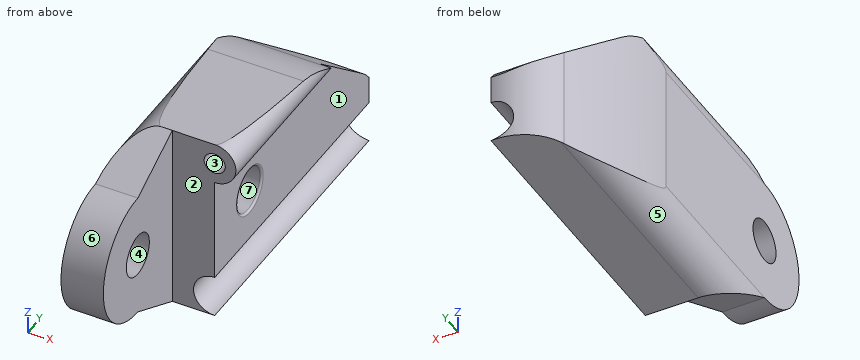
```python
from build123d import *

# Parameters (mm, degrees)
BOSS_EXTRUDE1_DEPTH = 50.8
CUT_EXTRUDE2_START  = -21.59
SKETCH3_R           = 1.27
CUT_EXTRUDE2_DEPTH  = 50.8
CUT_EXTRUDE1_DEPTH  = 50.8
SKETCH4_W           = 10.16
SKETCH4_H           = 15.24
CUT_EXTRUDE3_DEPTH  = 50.8
SKETCH5_R           = 2.54
CUT_EXTRUDE5_DEPTH  = 50.8
CUT_EXTRUDE6_DEPTH  = 32.512
CUT_EXTRUDE7_DEPTH  = 32.512
CUT_EXTRUDE12_START = -10.16
SKETCH14_R          = 2.7
CUT_EXTRUDE12_DEPTH = 9.08
CUT_EXTRUDE9_DEPTH  = 38.608
BOSS_EXTRUDE2_START = -4.2
SKETCH15_R          = 2.7
BOSS_EXTRUDE2_DEPTH = 4.2
FILLET1_R           = 0.254
SKETCH16_R          = 1.7526
CUT_EXTRUDE13_DEPTH = 3.556


with BuildPart() as part:
    # Sketch1 → Boss-Extrude1 (new body)
    with BuildSketch(Plane(origin=(0, 0, 0), x_dir=(1, 0, 0), z_dir=(0, 1, 0))):
        with BuildLine():
            Line((-20.32, 27.095319289), (-20.32, 11.855319289))
            ThreePointArc((-20.32, 11.855319289), (-19.204076836, 9.161242453), (-16.51, 8.045319289))
            Line((-16.51, 8.045319289), (-3.81, 8.045319289))
            ThreePointArc((-3.81, 8.045319289), (-1.115923164, 9.161242453), (0, 11.855319289))
            Line((0, 11.855319289), (0, 27.095319289))
            ThreePointArc((0, 27.095319289), (-1.115923164, 29.789396126), (-3.81, 30.905319289))
            Line((-3.81, 30.905319289), (-16.51, 30.905319289))
            ThreePointArc((-16.51, 30.905319289), (-19.204076836, 29.789396126), (-20.32, 27.095319289))
        make_face()
    extrude(amount=BOSS_EXTRUDE1_DEPTH)

    # Sketch3 → Cut-Extrude2 (cut)
    with BuildSketch(Plane(origin=(0, 50.8, 0), x_dir=(1, 0, 0), z_dir=(0, 1, 0)).offset(CUT_EXTRUDE2_START)):
        with Locations(Location((-10.16, 10.585319289, 0), (0, 0, 270))):
            Circle(SKETCH3_R)
        with Locations(Location((-10.16, 28.365319289, 0), (0, 0, 270))):
            Circle(SKETCH3_R)
    extrude(amount=-CUT_EXTRUDE2_DEPTH, mode=Mode.SUBTRACT)

    # Sketch2 → Cut-Extrude1 (cut)
    with BuildSketch(Plane.ZY.offset(20.32)):
        with BuildLine():
            Line((-27.095319289, 7.62), (-30.905319289, 15.24))
            Line((-30.905319289, 15.24), (-30.905319289, -5.08))
            Line((-30.905319289, -5.08), (-8.045319289, -5.08))
            Line((-8.045319289, -5.08), (-8.045319289, 15.24))
            Line((-8.045319289, 15.24), (-11.855319289, 7.62))
            ThreePointArc((-11.855319289, 7.62), (-19.475319289, 0), (-27.095319289, 7.62))
        make_face()
    extrude(amount=-CUT_EXTRUDE1_DEPTH, mode=Mode.SUBTRACT)

    # Sketch4 → Cut-Extrude3 (cut)
    with BuildSketch(Plane.XY.offset(-8.045319289)):
        with Locations((-10.16, 7.62)):
            Rectangle(SKETCH4_W, SKETCH4_H)
    extrude(amount=-CUT_EXTRUDE3_DEPTH, mode=Mode.SUBTRACT)

    # Sketch5 → Cut-Extrude5 (cut)
    with BuildSketch(Plane.ZY.offset(20.32)):
        with Locations((-19.475319289, 7.62)):
            Circle(SKETCH5_R)
    extrude(amount=-CUT_EXTRUDE5_DEPTH, mode=Mode.SUBTRACT)

    # Sketch6 → Cut-Extrude6 (cut)
    with BuildSketch(Plane.ZY.offset(20.32)):
        with BuildLine():
            Line((-11.855319289, 36.846817341), (-21.012334943, 47.93447962))
            ThreePointArc((-21.012334943, 47.93447962), (-23.733254983, 50.047756788), (-27.095319289, 50.8))
            Line((-27.095319289, 50.8), (-31.52544936, 50.8))
            Line((-31.52544936, 50.8), (-31.52544936, 15.08846866))
            Line((-31.52544936, 15.08846866), (-40.392656277, 51.934271372))
            Line((-40.392656277, 51.934271372), (12.273740193, 71.26134954))
            Line((12.273740193, 71.26134954), (-8.045319289, 15.24))
            Line((-8.045319289, 15.24), (-9.357524517, 30.725540243))
            ThreePointArc((-9.357524517, 30.725540243), (-10.139323425, 33.97677891), (-11.855319289, 36.846817341))
        make_face()
    extrude(amount=-CUT_EXTRUDE6_DEPTH, mode=Mode.SUBTRACT)

    # Sketch7 → Cut-Extrude7 (cut)
    with BuildSketch(Plane(origin=(0, 0, -30.905319289), x_dir=(-1, 0, 0), z_dir=(0, 0, -1))):
        with BuildLine():
            Line((0, 29.335182296), (-12.852337187, 67.804770192))
            Line((-12.852337187, 67.804770192), (37.594938904, 66.861563092))
            Line((37.594938904, 66.861563092), (20.32, 29.335182296))
            ThreePointArc((20.32, 29.335182296), (19.06442366, 37.382371637), (16.68228589, 45.170769925))
            ThreePointArc((16.68228589, 45.170769925), (10.662952429, 49.301878805), (4.643618968, 45.170769925))
            ThreePointArc((4.643618968, 45.170769925), (1.994617848, 37.348921605), (0, 29.335182296))
        make_face()
    extrude(amount=-CUT_EXTRUDE7_DEPTH, mode=Mode.SUBTRACT)

    # Sketch14 → Cut-Extrude12 (cut)
    with BuildSketch(Plane(origin=(0, 0, 0), x_dir=(0, 0, -1), z_dir=(1, 0, 0)).offset(CUT_EXTRUDE12_START)):
        with Locations((19.475319289, 22.985182296)):
            Circle(SKETCH14_R)
    extrude(amount=-CUT_EXTRUDE12_DEPTH, mode=Mode.SUBTRACT)

    # Sketch8 → Cut-Extrude9 (cut, symmetric)
    with BuildSketch(Plane.XZ.offset(-15.24)):
        with BuildLine():
            Line((-10.16, -13.125319289), (-10.16, -25.825319289))
            ThreePointArc((-10.16, -25.825319289), (-12.7, -28.365319289), (-10.16, -30.905319289))
            Line((-10.16, -30.905319289), (15.115555145, -54.006547143))
            Line((15.115555145, -54.006547143), (12.290345115, 18.720711385))
            Line((12.290345115, 18.720711385), (-10.16, -8.045319289))
            ThreePointArc((-10.16, -8.045319289), (-7.62, -10.585319289), (-10.16, -13.125319289))
        make_face()
    extrude(amount=CUT_EXTRUDE9_DEPTH, both=True, mode=Mode.SUBTRACT)

    # Sketch15 → Boss-Extrude2 (add)
    with BuildSketch(Plane.ZY.offset(20.32).offset(BOSS_EXTRUDE2_START)):
        with Locations((-19.475319289, 22.985182296)):
            Circle(SKETCH15_R)
    extrude(amount=BOSS_EXTRUDE2_DEPTH)

    # Fillet1
    fillet1_edges = [part.edges().sort_by_distance(p)[0] for p in [
        (-10.16, 22.985182296, -16.775319289),
    ]]
    fillet(fillet1_edges, radius=FILLET1_R)

    # Sketch16 → Cut-Extrude13 (cut)
    with BuildSketch(Plane(origin=(-16.12, 0, 0), x_dir=(0, 0, -1), z_dir=(1, 0, 0))):
        with Locations((19.475319289, 22.985182296)):
            Circle(SKETCH16_R)
    extrude(amount=-CUT_EXTRUDE13_DEPTH, mode=Mode.SUBTRACT)


solid = part.part
```
Read the model definition and answer for the solid it produces. Units are mm, in the model's axes. Face numbers are marked on the shaded views. A direction names the side the tool comes from. Give positions to 0.01 mm unless a question says otherwise; leave off trailing zeros. Order: outer loops, then holes, each group sorted by start corner. A loop starts at its lowest first (then second) coordinate and runs counter-clockwise, first axis right, second up. Notation, with made-up numbers: (86, 27.5) -> (114, 27.5) arc R9 cw to (114, 32.5) -> close; hole circle Ø3 at (-23.5, 64). An arc over 180 degrees is marked (long way). Write item = value, one per line.
1. A cutting plane is placed at C-C, the plane z = -23.25. Write down the section's boundary in (x, y), and give its area (3 significant figures).
Numbers:
outline = (-20.32, 1) -> (-15.24, 1) -> (-15.24, 15.24) -> (-10.16, 15.24) -> (-10.16, 49.28) arc R6.45 ccw to (-16.68, 45.17) arc R57.39 ccw to (-20.32, 29.34) -> close
area = 374 mm²
2. Straight lines are drawn through the part: line 1 along X through (y, z) = (24, -15.75); line 2 along Y through (x, z) = (-12.5, -19.75); line 3 along Z through (x, y) = (-14.75, 34). For each, find the intervals that lie inside material, in ascending order.
Numbers:
line_1 = -20.32 to -10.16
line_2 = 15.24 to 20.3, 25.67 to 46.41
line_3 = -30.91 to -10.15
3. A cutting plane is placed at D-D, the plane y = 35. Write down the section's boundary in (x, z), and give its area (3 significant figures).
Numbers:
outline = (-19.56, -29.38) arc R3.81 ccw to (-16.51, -30.91) -> (-10.16, -30.91) arc R2.54 cw to (-10.16, -25.83) -> (-10.16, -13.13) arc R2.54 ccw to (-7.62, -10.62) -> (-19.56, -10.62) -> close
area = 184 mm²
4. Given pin 1 (5 mm diameter, centred on y = 20, z = -15, fed in from +X); pin 2 (4 mm diameter, centred on y = 22.99, z = -19.48, fed in from +X); pin 3 (3 mm diameter, centred on x = -10.16, z = -10.59, fed in from +Y); pin 4 (1.5 mm diameter, centred on x = -12, y = 12.5, fed in from +Z), each flat-ended and moving along its own axis, determine where each tip first touches the part or whether it passes through.
Numbers:
pin_1 = -8.49
pin_2 = -16.12
pin_3 = 37.13
pin_4 = through
5. For the marked faces 1, 2 and 3, determine the directions among +Z, -Z, +X, -X, +Y, -Y from which every point of the face is accessible in a straight line to the end or side of a thin tool.
Numbers:
face_1 = -Z, +X, +Y, -Y
face_2 = +Z, -Z, +X, -Y
face_3 = -Y
6. The mould has two halves that part along Z. Classify the marked faces 4, 5, 6 and 7: +Z half, -Z half, draft (parallel to the pull), parting line (faces both ways), or undercut.
Numbers:
face_4 = undercut
face_5 = -Z half
face_6 = parting line
face_7 = undercut
7. A cutting plane is placed at A-A, the plane y = 8.5. Write down the section's boundary in (x, z), and give its area (3 significant figures).
Numbers:
outline = (-20.32, -27.1) arc R3.81 ccw to (-20.29, -27.54) -> (-15.24, -27.54) -> (-15.24, -21.86) -> (-20.32, -21.86) -> close; (-20.32, -17.09) -> (-15.24, -17.09) -> (-15.24, -11.42) -> (-20.29, -11.42) arc R3.81 ccw to (-20.32, -11.86) -> close
area = 57.7 mm²
8. A cutting plane is placed at B-B, the plane y = 17.5. Write down the section's boundary in (x, z).
Numbers:
outline = (-20.32, -27.1) arc R3.81 ccw to (-16.51, -30.91) -> (-10.16, -30.91) arc R2.54 cw to (-10.16, -25.83) -> (-10.16, -13.13) arc R2.54 ccw to (-9.19, -8.24) -> (-17.7, -8.24) arc R3.81 ccw to (-20.32, -11.86) -> close; hole circle Ø2.54 at (-10.16, -10.59)
